from build123d import *

# Parameters (mm, degrees)
SKETCH1_W                  = 155
SKETCH1_H                  = 30
BOSS_EXTRUDE1_DEPTH        = 17.5
FILLET1_R                  = 5
M4_TAPPED_HOLE2_AT_2_COUNT = 2
M4_TAPPED_HOLE2_AT_2_PITCH = 60
M4_TAPPED_HOLE2_AT_3_COUNT = 2
M4_TAPPED_HOLE2_AT_3_PITCH = 175.570498661
M4_TAPPED_HOLE2_AT_4_COUNT = 2
M4_TAPPED_HOLE2_AT_4_PITCH = 165


with BuildPart() as part:
    # Sketch1 → Boss-Extrude1 (new, symmetric)
    with BuildSketch(Plane(origin=(0, 0, 0), x_dir=(1, 0, 0), z_dir=(0, 1, 0))):
        Polygon((-87.5, 25), (87.5, 25), (87.5, -25), (87.5, -85), (77.5, -85), (77.5, -25), (-77.5, -25), (-77.5, -85), (-87.5, -85), (-87.5, -25), align=None)
        Rectangle(SKETCH1_W, SKETCH1_H, mode=Mode.SUBTRACT)
    extrude(amount=BOSS_EXTRUDE1_DEPTH, both=True)

    # Fillet1
    fillet1_edges = [part.edges().sort_by_distance(p)[0] for p in [
        (77.5, 0, 25),
        (-77.5, 0, 25),
        (-77.5, 0, 15),
        (-77.5, 0, -15),
        (77.5, 0, -15),
        (77.5, 0, 15),
    ]]
    fillet(fillet1_edges, radius=FILLET1_R)

    # Sketch4 → M4 Tapped Hole2 (revolve, cut)
    with BuildSketch(Plane(origin=(-82.5, 17.5, 20), x_dir=(0, 0, 1), z_dir=(1, 0, 0))):
        Polygon((0, 0), (0, 16.991420021), (1.65, 16), (1.65, 0), align=None)
    m4_tapped_hole2 = revolve(axis=Axis((-82.5, 23.85, 20), (0, -1, 0)), mode=Mode.SUBTRACT)

    # M4 Tapped Hole2 at 2: M4 Tapped Hole2 ×2
    with Locations(*[(0, 0, i * M4_TAPPED_HOLE2_AT_2_PITCH) for i in range(1, M4_TAPPED_HOLE2_AT_2_COUNT)]):
        add(m4_tapped_hole2, mode=Mode.SUBTRACT)

    # M4 Tapped Hole2 at 3: M4 Tapped Hole2 ×2
    with Locations(*[Vector(0.9397934234884371, 0, 0.3417430630867045) * (i * M4_TAPPED_HOLE2_AT_3_PITCH) for i in range(1, M4_TAPPED_HOLE2_AT_3_COUNT)]):
        add(m4_tapped_hole2, mode=Mode.SUBTRACT)

    # M4 Tapped Hole2 at 4: M4 Tapped Hole2 ×2
    with Locations(*[(i * M4_TAPPED_HOLE2_AT_4_PITCH, 0, 0) for i in range(1, M4_TAPPED_HOLE2_AT_4_COUNT)]):
        add(m4_tapped_hole2, mode=Mode.SUBTRACT)

    # Mirror1: M4 Tapped Hole2 across plane
    add(m4_tapped_hole2.mirror(Plane.ZX), mode=Mode.SUBTRACT)

    # Mirror1 copy 1 sketch → Mirror1 copy 1 (revolve, cut)
    with BuildSketch(Plane(origin=(-82.5, -17.5, 80), x_dir=(0, 0, 1), z_dir=(1, 0, 0))):
        Polygon((0, 0), (0, -16.991420021), (1.65, -16), (1.65, 0), align=None)
    revolve(axis=Axis((-82.5, -23.85, 80), (0, -1, 0)), mode=Mode.SUBTRACT)

    # Mirror1 copy 2 sketch → Mirror1 copy 2 (revolve, cut)
    with BuildSketch(Plane(origin=(82.5, -17.5, 80), x_dir=(0, 0, 1), z_dir=(1, 0, 0))):
        Polygon((0, 0), (0, -16.991420021), (1.65, -16), (1.65, 0), align=None)
    revolve(axis=Axis((82.5, -23.85, 80), (0, -1, 0)), mode=Mode.SUBTRACT)

    # Mirror1 copy 3 sketch → Mirror1 copy 3 (revolve, cut)
    with BuildSketch(Plane(origin=(82.5, -17.5, 20), x_dir=(0, 0, 1), z_dir=(1, 0, 0))):
        Polygon((0, 0), (0, -16.991420021), (1.65, -16), (1.65, 0), align=None)
    revolve(axis=Axis((82.5, -23.85, 20), (0, -1, 0)), mode=Mode.SUBTRACT)


solid = part.part
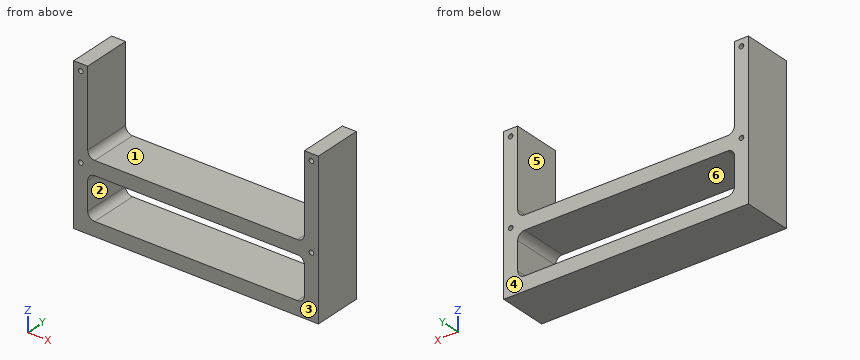
Work out the finished part from the listing and answer in its coordinate system (mm). Face numbers are marked on the shaded views. A direction names the side the tool comes from. Coordinates: 2 decimals unless noted, no trailing zeros. Loops run counter-clockwise (first coordinate to the right, second up) from the corner with the lowest first, then second, coordinate; pieces in that order, holes last. Notation, with made-up numbers: M 14,-36 L 26,-36 A24 ccw 26,-21 Z; hole C 16,-24.5 d1. An arc over 180 degrees is marked long. Answer in a Markdown table with one row per item. Add a question column.
1. Find section B-B, the plane z = 73.5. Write down the section's boundary in (x, y).
2. A tool of negligible diameter and unlimited length cuts with its end or side. For the marked faces 4, 5 and 6, from which of +Z, -Z, +X, -X, +Y, -Y can it reach the whole face along a straight path? Write none if from no direction.
3. The mould has two halves that part along Z. Classify the marked faces 1, 2 and 3: pulls with the +Z half, pulls with the -Z half, needs draft (parallel to the pull), parting line crosses it, or undercut.
4. Find section C-C, the plane y = -6.5. Write down the section's boundary in (x, z).
5. Flat-ended cylindrical pins translate along their axes: P1, Ø3, axis at x = -82.5, z = 80, coming from the -Y side; P2, Ø8, axis at x = -49.5, y = 1.5, coming from the +Z side; P3, Ø2.5, axis at x = -82.5, z = 20, coming from the +Y side. Find the tip coordinate at first contact, or state that the pin passes through.
6. Find section A-A, the plane x = 27.5. Write down the section's boundary in (y, z).
7. Consider L1, parallel to Z at x = -82.5, y = 9.75; L2, parallel to X at y = -10, z = 20; L3, parallel to Z at x = 38, y = -4.5. Determine where each line is inside the solid, lowest interval first.
Reported:
| question | item | result |
|---|---|---|
| 1 | outline | M -87.5,-17.5 L -77.5,-17.5 L -77.5,17.5 L -87.5,17.5 Z; M 77.5,-17.5 L 87.5,-17.5 L 87.5,17.5 L 77.5,17.5 Z |
| 2 | face 4 | +Z, -Z, +X, -X, +Y |
| 2 | face 5 | +Z, +Y, -Y |
| 2 | face 6 | +Y, -Y |
| 3 | face 1 | pulls with the +Z half |
| 3 | face 2 | undercut |
| 3 | face 3 | needs draft |
| 4 | outline | M -87.5,-25 L 87.5,-25 L 87.5,85 L 77.5,85 L 77.5,30 A5 cw 72.5,25 L -72.5,25 A5 cw -77.5,30 L -77.5,85 L -87.5,85 Z; hole C -82.5,20 d3.3; hole C -82.5,80 d3.3; hole M -77.5,-10 A5 ccw -72.5,-15 L 72.5,-15 A5 ccw 77.5,-10 L 77.5,10 A5 ccw 72.5,15 L -72.5,15 A5 ccw -77.5,10 Z; hole C 82.5,20 d3.3; hole C 82.5,80 d3.3 |
| 5 | P1 | stops at y = -1.41 |
| 5 | P2 | stops at z = 25 |
| 5 | P3 | stops at y = 1.26 |
| 6 | outline | M -17.5,-25 L 17.5,-25 L 17.5,-15 L -17.5,-15 Z; M -17.5,15 L 17.5,15 L 17.5,25 L -17.5,25 Z |
| 7 | L1 | z = -25 to 18.35, 21.65 to 78.35, 81.65 to 85 |
| 7 | L2 | x = -87.5 to -84.15, -80.85 to 80.85, 84.15 to 87.5 |
| 7 | L3 | z = -25 to -15, 15 to 25 |
